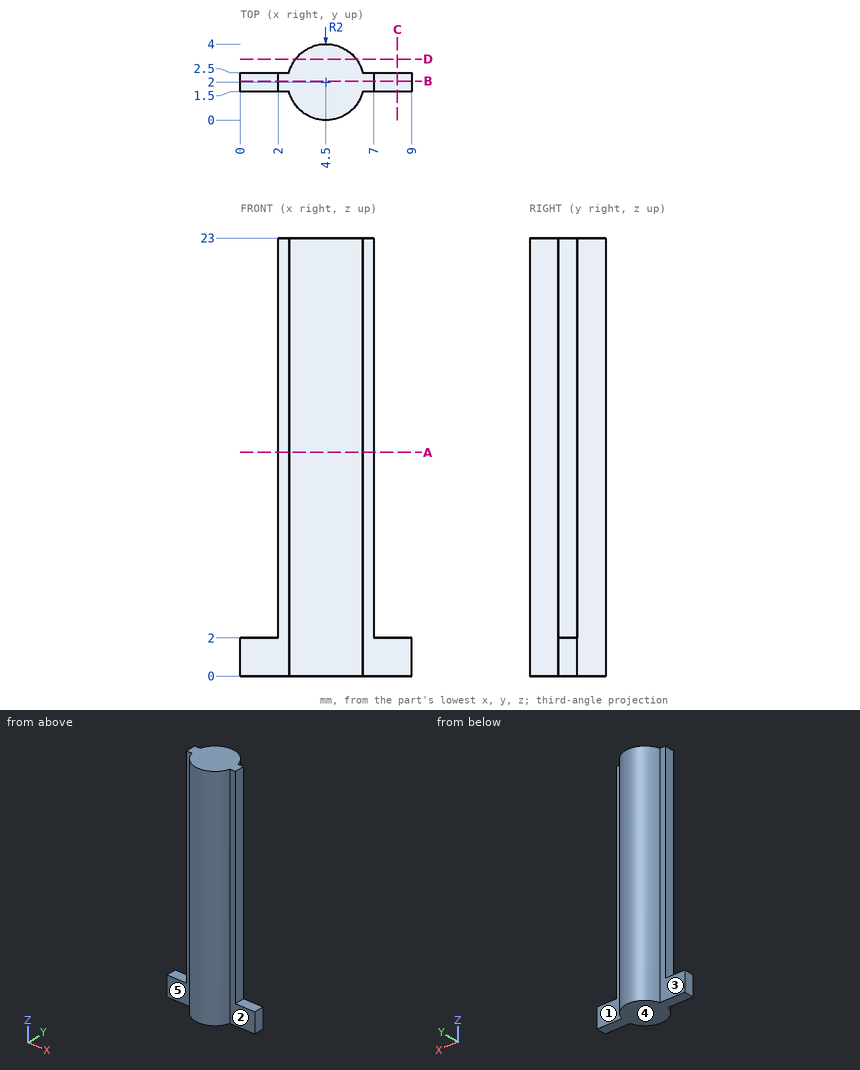
Input: dimensioned drawing with shaded views. Units: mm. Origin: part minimum x, y, z. A direction names the side the tool comes from. Give positions to 0.01 mm unless a question says otherwise; leave off trailing zeros. Write each loop counter-clockwise with the first axis right and the second up, starting at its lowest first coordinate (ties: lowest second). Pieces come first, ordered by that corner, then holes. Notation, with made-up numbers: (-8.5, 7) - (48.5, 7) arc R28 cw to (48.5, 32) - close; hole circle Ø2 at (-18.75, -29). An arc over 180 degrees is marked (long way). Write item = value, one per line. Start each with the question number.
1) Material intervals for L1, parallel to Y at x = 6.5, z = 16.25; L2, parallel to X at y = 2.3, z = 12.75; L3, parallel to X at y = 0.4, z = 18.5, sorted ascending. Write a range as [from, to].
2) Cut plane B-B (y = 2.05). Return loops of the section in (x, z).
3) Reachability of the marked faces 1, 2, 3, 4 and 5 from +Z, -Z, +X, -X, +Y, -Y: full face, straight path, thin tool, end or side. Return the list, or none.
4) Cut plane C-C (x = 8.25). Return loops of the section in (y, z).
5) Cut plane A-A (z = 11.75). Return loops of the section in (x, y).
6) Pin query (flat end, axial travel): pin 1 (2 mm diameter, centred on y = 2, z = 7.5, fed in from +X); pin 2 (1 mm diameter, centred on y = 3.5, z = 15.5, fed in from -X); pin 3 (0.8 mm diameter, centred on x = 1.5, y = 2, fed in from +Z). Return the tip coordinate at first contact, or that it passes through.
7) Cut plane D-D (y = 3.2). Return loops of the section in (x, z), and give its area (3 significant figures).
Answers follow:
q1.L1 = [1.5, 2.5]
q1.L2 = [2, 7]
q1.L3 = [3.3, 5.7]
q2.outline = (0, 0) - (9, 0) - (9, 2) - (7, 2) - (7, 23) - (2, 23) - (2, 2) - (0, 2) - close
q3.face_1 = +Z, -Z, +X, +Y
q3.face_2 = +Z, -Z, +X, -Y
q3.face_3 = +Z, -Z, -X, +Y
q3.face_4 = -Z, +X, -X, +Y, -Y
q3.face_5 = +Z, -Z, -X, -Y
q4.outline = (1.5, 0) - (2.5, 0) - (2.5, 2) - (1.5, 2) - close
q5.outline = (2, 1.5) - (2.56, 1.5) arc R2 ccw to (6.44, 1.5) - (7, 1.5) - (7, 2.5) - (6.44, 2.5) arc R2 ccw to (2.56, 2.5) - (2, 2.5) - close
q6.pin_1 = 7
q6.pin_2 = 2.77
q6.pin_3 = 2
q7.outline = (2.9, 0) - (6.1, 0) - (6.1, 23) - (2.9, 23) - close
q7.area = 73.6 mm^2
